from build123d import *

# Parameters (mm, degrees)
F1_DEPTH    = 6.35
F2_T1_DEPTH = 6.35
F3_R        = 1.27


# Not quite as in the source:
# - a fillet or chamfer that OpenCascade refuses, or shapes differently, is made with other operations: its cross-section is extruded or revolved along the edge and cut away or added


with BuildPart() as f1:
    # F0 (on Top) → F1 (new body)
    with BuildSketch(Plane.XY):
        Polygon((28.2575, 0), (0, 0), (0, -4.7625), (39.37, -4.7625), (39.37, -12.3825), (44.1325, -12.3825), (44.1325, 0), (37.7825, 0), (37.7825, 3.175), (36.195, 3.175), (36.195, 0), (29.845, 0), (29.845, 3.175), (28.2575, 3.175), align=None)
    extrude(amount=F1_DEPTH)

    # F2: fillet of radius 5.08 on 2 edges, made by hand

    # F2_s2 → F2_t1 (join)
    with BuildSketch(Plane.XY):
        with BuildLine():
            ThreePointArc((42.4917860393, 0), (39.6519797079, 0.8678865162), (37.7825, 3.175))
            Line((37.7825, 3.175), (37.7825, 0))
            Line((37.7825, 0), (42.4917860393, 0))
        make_face()
        with BuildLine():
            ThreePointArc((23.5482139607, 0), (26.3880202921, 0.8678865162), (28.2575, 3.175))
            Line((28.2575, 3.175), (28.2575, 0))
            Line((28.2575, 0), (23.5482139607, 0))
        make_face()
    extrude(amount=F2_T1_DEPTH)

    # F3
    f3_edges = [f1.edges().sort_by_distance(p)[0] for p in [
        (39.37, -8.5725, 0),
        (44.1325, -6.19125, 6.35),
        (41.75125, -12.3825, 6.35),
        (44.1325, -12.3825, 3.175),
        (39.37, -12.3825, 3.175),
        (41.75125, -12.3825, 0),
        (39.37, -8.5725, 6.35),
        (44.1325, -6.19125, 0),
        (39.65198, 0.867887, 6.35),
        (39.65198, 0.867887, 0),
        (43.312143, 0, 6.35),
        (43.312143, 0, 0),
        (44.1325, 0, 3.175),
    ]]
    fillet(f3_edges, radius=F3_R)

    # F4: F1 across plane


with BuildPart() as f1_1:
    add(f1.part)
    add(f1.part.mirror(Plane.YZ))


solid = f1_1.part
Part model, mm, in its own coordinate system. A direction names the side the tool comes from. Give positions to 0.01 mm unless a question says otherwise; leave off trailing zeros. Order: outer loops, then holes, each group sorted by start corner. A loop starts at its lowest first (then second) coordinate and runs counter-clockwise, first axis right, second up. Notation, with made-up numbers: (-10.5, 51.25) - (31.5, 51.25) arc R25 cw to (31.5, 68.25) - close; hole circle Ø6 at (46, 10.25). An arc over 180 degrees is marked (long way). Use a Markdown table: item, result.
1) Saw through at D-D on y = 1.25. Count the separate pieces of the cut face and the enclosed holes in it, plus the area to 3 significant figures.
Checked values:
| item | result |
|---|---|
| separate pieces | 4 |
| enclosed holes | 0 |
| area | 73.2 mm² |
2) Two-plate mould, pull along X, no slides. Class faces 4 (the flat face through (37, 3.175, 3)), 5 (the flat face through (29.845, 2, 3)), 6 (the flat face through (44.132, -6, 3)): +X half, -X half, draft (parallel to the pull), parting line (faces both ways), or undercut.
Checked values:
| item | result |
|---|---|
| face 4 | draft |
| face 5 | undercut |
| face 6 | +X half |
3) Saw through at C-C on x = 22. List the corners of the cut face in (y, z), plus the area to 3 significant figures.
Checked values:
| item | result |
|---|---|
| outline | (-4.76, 0) - (0, 0) - (0, 6.35) - (-4.76, 6.35) - close |
| area | 30.2 mm² |
4) Probe L1, parallel to X at y = -5, z = 4.5; L2, parallel to Y at x = -20.5, z = 4.5; L3, parallel to X at y = -4, z = 5.25. List the from-to ranges inside material, lowest first. Write a range as from..to.
Checked values:
| item | result |
|---|---|
| L1 | -44.13..-39.37, 39.37..44.13 |
| L2 | -4.76..0 |
| L3 | -44.12..44.12 |
5) 3-axis set-ups, long thin cutter, end or side, ignore diameter. For faces 1 (the flat face through (42, -12.382, 3)), 2 (the flat face through (36.195, 2, 3)), 3 (the flat face through (39.37, -8, 3)): which of +Z, -Z, +X, -X, +Y, -Y reach the whole face in a straight line?
Checked values:
| item | result |
|---|---|
| face 1 | +Z, -Z, +X, -X, -Y |
| face 2 | +Z, -Z, +Y |
| face 3 | +Z, -Z, -Y |
6) Flat gauge pins, fed straight in: P1, Ø3.5, axis at y = 1, z = 3, coming from the -X side; P2, Ø1, axis at x = -24.5, z = 2, coming from the -Y side; P3, Ø1, axis at y = 2.5, z = 4, coming from the +X side. Where does each tip first touch, or does it go through?
Checked values:
| item | result |
|---|---|
| P1 | x = -44.02 |
| P2 | y = -4.76 |
| P3 | x = 38.45 |
7) Saw through at A-A on y = -7. List the corners of the cut face in (x, z).
Checked values:
| item | result |
|---|---|
| outline | (-44.13, 1.27) arc R1.27 ccw to (-42.86, 0) - (-40.64, 0) arc R1.27 ccw to (-39.37, 1.27) - (-39.37, 5.08) arc R1.27 ccw to (-40.64, 6.35) - (-42.86, 6.35) arc R1.27 ccw to (-44.13, 5.08) - close; (39.37, 1.27) arc R1.27 ccw to (40.64, 0) - (42.86, 0) arc R1.27 ccw to (44.13, 1.27) - (44.13, 5.08) arc R1.27 ccw to (42.86, 6.35) - (40.64, 6.35) arc R1.27 ccw to (39.37, 5.08) - close |
